Geometry: final body of the model. Coordinates: model frame, mm. Face numbers are marked on the shaded views. A direction names the side the tool comes from. Coordinates: 2 decimals unless noted, no trailing zeros. Loops run counter-clockwise (first coordinate to the right, second up) from the corner with the lowest first, then second, coordinate; pieces in that order, holes last. Notation, with made-up numbers: (30.5, -27.75) - (44.5, -27.75) arc R18 ccw to (44.5, -9.75) - close; hole circle Ø10 at (-36.5, 0). An arc over 180 degrees is marked (long way). Answer in a Markdown table with one row per item.
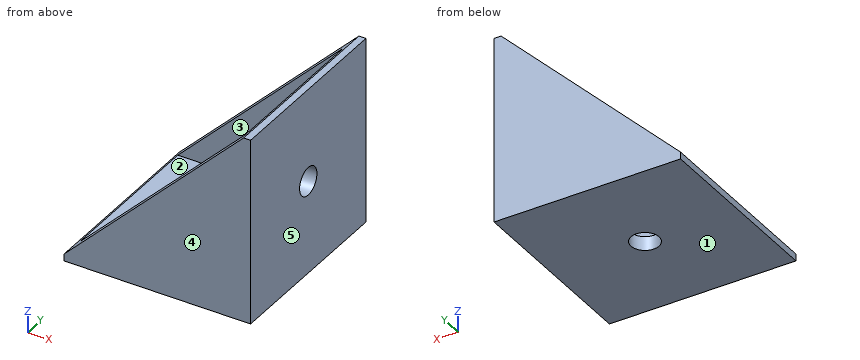
from build123d import *

# Parameters (mm, degrees)
BOSS_EXTRUDE1_DEPTH = 20
SKETCH3_R           = 3
CUT_EXTRUDE1_DEPTH  = 20
SKETCH4_R           = 3
CUT_EXTRUDE2_DEPTH  = 20
BOSS_EXTRUDE2_DEPTH = 3


with BuildPart() as part:
    # Sketch2 → Boss-Extrude1 (new body, symmetric)
    with BuildSketch(Plane(origin=(0, 0, 0), x_dir=(1, 0, 0), z_dir=(0, 1, 0))):
        Polygon((0, 0), (-40, 0), (-40, -1.5), (-38.5, -3), (-3, -3), (-3, -38.5), (-1.5, -40), (0, -40), align=None)
    extrude(amount=BOSS_EXTRUDE1_DEPTH, both=True)

    # Sketch3 → Cut-Extrude1 (cut, symmetric)
    with BuildSketch(Plane.XY.offset(3)):
        with Locations((-20, 0)):
            Circle(SKETCH3_R)
    extrude(amount=CUT_EXTRUDE1_DEPTH, both=True, mode=Mode.SUBTRACT)

    # Sketch4 → Cut-Extrude2 (cut, symmetric)
    with BuildSketch(Plane.ZY.offset(3)):
        with Locations((20, 0)):
            Circle(SKETCH4_R)
    extrude(amount=CUT_EXTRUDE2_DEPTH, both=True, mode=Mode.SUBTRACT)

    # Sketch5 → Boss-Extrude2 (add)
    with BuildSketch(Plane.XZ.offset(20)):
        Polygon((-38.5, 3), (-3, 38.5), (-3, 3), align=None)
    boss_extrude2 = extrude(amount=-BOSS_EXTRUDE2_DEPTH)

    # Mirror1: Boss-Extrude2 across plane
    add(boss_extrude2.mirror(Plane.ZX))


solid = part.part
(1) Cut plane C-C on x = -20. Output: boundary loops of the cut face in (y, z).
Verdict:
| item | result |
|---|---|
| outline | (-20, 0) - (-3, 0) - (-3, 3) - (-17, 3) - (-17, 21.5) - (-20, 21.5) - close; (3, 0) - (20, 0) - (20, 21.5) - (17, 21.5) - (17, 3) - (3, 3) - close |
(2) Ray query, probe 1 along Y at (x, z) = (-7, 30); probe 2 along Y at (x, z) = (-0.7, 20); probe 3 along Z at (x, y) = (-9, 3). Return the intervals inside material, ascending.
Verdict:
| item | result |
|---|---|
| probe 1 | y = -20 to -17, 17 to 20 |
| probe 2 | y = -20 to -3, 3 to 20 |
| probe 3 | z = 0 to 3 |
(3) First-contact query: pin 1 Ø12 at (y, z) = (15, 8) entering from -X; pin 2 Ø2 at (x, y) = (-33.5, 9) entering from +Z; pin 3 Ø5.5 at (x, y) = (-20, 0) entering from -Z; pin 4 Ø10 at (y, z) = (1.5, 25) entering from -X. Flat tips, straight axial feed; report the tip coordinate or a pass-through.
Verdict:
| item | result |
|---|---|
| pin 1 | stops at x = -39.5 |
| pin 2 | stops at z = 3 |
| pin 3 | passes through |
| pin 4 | stops at x = -3 |
(4) Access query for the marked faces 1 and 2. Directions: +Z, -Z, +X, -X, +Y, -Y. A direction counts if a zero-diameter tool reaches every point of the face in a straight line with its end or side. Return the directions, or none.
Verdict:
| item | result |
|---|---|
| face 1 | -Z, +X, -X, +Y, -Y |
| face 2 | +Z, -X |
(5) Cut plane B-B on z = 20. Output: boundary loops of the cut face in (x, y), then the cut area to 3 significant figures.
Verdict:
| item | result |
|---|---|
| outline | (-21.5, -20) - (0, -20) - (0, -3) - (-3, -3) - (-3, -17) - (-21.5, -17) - close; (-21.5, 17) - (-3, 17) - (-3, 3) - (0, 3) - (0, 20) - (-21.5, 20) - close |
| area | 213 mm² |
(6) Pull-direction query (Y, two-part tool) for the marked faces 3, 4 and 5; classes: pulls with the +Y half, pulls with the -Y half, needs draft (parallel to the pull), parting line crosses it, or undercut.
Verdict:
| item | result |
|---|---|
| face 3 | undercut |
| face 4 | pulls with the -Y half |
| face 5 | needs draft |
(7) Cut plane D-D on z = 7.5. Output: boundary loops of the cut face in (x, y), then the cut area to 3 significant figures.
Verdict:
| item | result |
|---|---|
| outline | (-34, -20) - (0, -20) - (0, 20) - (-34, 20) - (-34, 17) - (-3, 17) - (-3, -17) - (-34, -17) - close |
| area | 306 mm² |
(8) Cut plane A-A on y = 0. Output: boundary loops of the cut face in (x, z).
Verdict:
| item | result |
|---|---|
| outline | (-40, 0) - (-23, 0) - (-23, 3) - (-38.5, 3) - (-40, 1.5) - close; (-17, 0) - (0, 0) - (0, 17) - (-3, 17) - (-3, 3) - (-17, 3) - close; (-3, 23) - (0, 23) - (0, 40) - (-1.5, 40) - (-3, 38.5) - close |
